Geometry: final body of the model. Coordinates: model frame, mm. A direction names the side the tool comes from. Give positions to 0.01 mm unless a question says otherwise; leave off trailing zeros. Loops run counter-clockwise (first coordinate to the right, second up) from the corner with the lowest first, then second, coordinate; pieces in that order, holes last. Notation, with made-up numbers: (18, 56) - (29, 56) arc R7 cw to (29, 65) - close; hole circle Ø9 at (23, -5). An arc over 180 degrees is marked (long way). Use one line per item in the form item = value.
```python
from build123d import *

# Parameters (mm, degrees)
SKETCH1_R             = 2.794
BOSS_EXTRUDE1_DEPTH   = 10
BOSS_EXTRUDE1_2_DEPTH = 10
BOSS_EXTRUDE1_3_DEPTH = 10
SKETCH2_W             = 10.16
SKETCH2_H             = 30.16
BOSS_EXTRUDE2_DEPTH   = 82.55
BOSS_EXTRUDE3_START   = 10
SKETCH3_R             = 2.794
BOSS_EXTRUDE3_DEPTH   = 10


with BuildPart() as part:
    # Sketch1 → Boss-Extrude1 (new body)
    with BuildSketch(Plane.XY):
        with Locations((110, 20)):
            Circle(SKETCH1_R)
    extrude(amount=-BOSS_EXTRUDE1_DEPTH)



with BuildPart() as body_2:
    # Sketch1 → Boss-Extrude1 2 (new body)
    with BuildSketch(Plane.XY):
        with Locations((110, 10)):
            Circle(SKETCH1_R)
    extrude(amount=-BOSS_EXTRUDE1_2_DEPTH)


with BuildPart() as body_3:
    # Sketch1 → Boss-Extrude1 3 (new body)
    with BuildSketch(Plane.XY):
        with Locations((110, 30)):
            Circle(SKETCH1_R)
    extrude(amount=-BOSS_EXTRUDE1_3_DEPTH)


with BuildPart() as part_1:
    add(part.part)

    add(body_2.part)  # Boss-Extrude2 merges body 2

    add(body_3.part)  # Boss-Extrude2 merges body 3
    # Sketch2 → Boss-Extrude2 (add)
    with BuildSketch(Plane.XY):
        with Locations((110, 20)):
            Rectangle(SKETCH2_W, SKETCH2_H)
    extrude(amount=BOSS_EXTRUDE2_DEPTH)

    # Sketch3 → Boss-Extrude3 (add)
    with BuildSketch(Plane.XY.offset(82.55).offset(BOSS_EXTRUDE3_START)):
        with Locations((110, 10)):
            Circle(SKETCH3_R)
        with Locations((110, 20)):
            Circle(SKETCH3_R)
        with Locations((110, 30)):
            Circle(SKETCH3_R)
    extrude(amount=-BOSS_EXTRUDE3_DEPTH)


solid = part_1.part
```
(1) Pull-direction query (Y, two-part tool) for faces 4 (the face through (104.92, 20, 41)), 5 (the face through (107.94, 21.89, -4.93)), 6 (the face through (110, 35.08, 41)), 7 (the face through (110, 4.92, 41)); classes: released by +Y, released by -Y, zero draft, split by the parting line, or undercut.
Solution:
face_4 = zero draft
face_5 = undercut
face_6 = released by +Y
face_7 = released by -Y
(2) Cut plane B-B (x = 110). Return the cut outline in (y, z).
Solution:
outline = (4.92, 0) - (7.21, 0) - (7.21, -10) - (12.79, -10) - (12.79, 0) - (17.21, 0) - (17.21, -10) - (22.79, -10) - (22.79, 0) - (27.21, 0) - (27.21, -10) - (32.79, -10) - (32.79, 0) - (35.08, 0) - (35.08, 82.55) - (32.79, 82.55) - (32.79, 92.55) - (27.21, 92.55) - (27.21, 82.55) - (22.79, 82.55) - (22.79, 92.55) - (17.21, 92.55) - (17.21, 82.55) - (12.79, 82.55) - (12.79, 92.55) - (7.21, 92.55) - (7.21, 82.55) - (4.92, 82.55) - close
(3) Access query for faces 1 (the face through (110, 30, 92.55)), 2 (the face through (107.783, 8.3, -4.93)), 3 (the face through (107.94, 31.89, 87.62)). Directions: +Z, -Z, +X, -X, +Y, -Y. A direction counts if a zero-diameter tool reaches every point of the face in a straight line with its end or side. Return the directions, or none.
Solution:
face_1 = +Z, +X, -X, +Y, -Y
face_2 = -Z
face_3 = +Z
(4) Cut plane A-A (y = 30). Return the cut outline in (x, z), plus the area to 3 significant figures.
Solution:
outline = (104.92, 0) - (107.21, 0) - (107.21, -10) - (112.79, -10) - (112.79, 0) - (115.08, 0) - (115.08, 82.55) - (112.79, 82.55) - (112.79, 92.55) - (107.21, 92.55) - (107.21, 82.55) - (104.92, 82.55) - close
area = 950 mm2
(5) Pin query (flat end, axial travel): P1, Ø6, axis at x = 107.5, y = 11.5, coming from the +Z side. Return the tip coordinate at first contact, or that it passes through.
Solution:
P1 = 92.55
(6) Material intervals for L1, parallel to Y at x = 110.5, z = -4.5; L2, parallel to Z at x = 106.25, y = 9; L3, parallel to X at y = 32, z = -5, sorted ascending. Write a range as from..to.
Solution:
L1 = 7.25..12.75, 17.25..22.75, 27.25..32.75
L2 = 0..82.55
L3 = 108.05..111.95
